Source: CAD feature listing. Evaluate the final solid. Frame: model axes, mm. Round coordinates to 2 decimals unless told otherwise and drop trailing zeros. Loops run counter-clockwise (first coordinate to the right, second up) from the corner with the lowest first, then second, coordinate; pieces in that order, holes last. Notation, with made-up numbers: (-22.5, -14.5) - (34.5, -14.5) arc R13 cw to (34.5, 1.5) - close; hole circle Ø7 at (41, 2). An arc over 180 degrees is marked (long way). One line per question, with ' | ' between items. Start each with the question number.
1. Ray query, line 1 (X direction, y = 303, z = 6.75); line 2 (X direction, y = 427.5, z = 3.2); line 3 (Y direction, x = 309, z = 9.5). Return the intervals inside material, ascending.
2. Cut plane B-B (y = 55). Return loops of the section in (x, z).
3. Pin query (flat end, axial travel): pin 1 (5 mm diameter, centred on y = 187, z = 4.5, fed in from +X); pin 2 (4 mm diameter, centred on x = 111, y = 303, fed in from -Z); pin 3 (3 mm diameter, centred on y = 393.5, z = 6, fed in from +X); pin 4 (2.5 mm diameter, centred on x = 314, z = 7, fed in from +Y). Return the tip coordinate at first contact, or that it passes through.
4. Cut plane D-D (z = 2.5). Return loops of the section in (x, y).
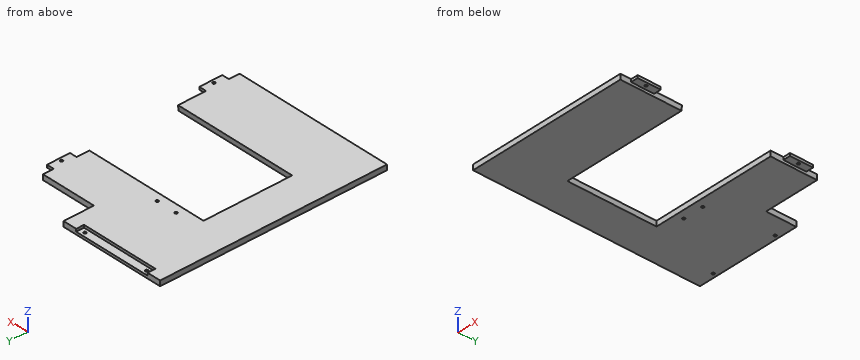
Autodesk Inventor part; units mm, degrees
ref_plane "YZ Plane" through (0, 0, 0) normal (1, 0, 0) x (0, 1, 0)
ref_plane "XZ Plane" through (0, 0, 0) normal (0, 1, 0) x (-1, 0, 0)
ref_plane "XY Plane" through (0, 0, 0) normal (0, 0, 1) x (1, 0, 0)
sketch "Sketch1" plane through (0, 0, 0) normal (0, 0, 1) x (1, 0, 0)
  line L0 (0, 0) -> (620, 0)
  line L1 (620, 0) -> (620, 620)
  line L2 (620, 620) -> (0, 620)
  line L3 (0, 620) -> (0, 0)
  line L4 (203, 491) -> (417, 491)
  line L5 (417, 491) -> (417, 377)
  line L6 (417, 377) -> (203, 377)
  line L7 (203, 377) -> (203, 491)
  point P0 (310, 491)
  point P1 (310, 620)
  dimension "d0" = 620
  dimension "d1" = 620
  dimension "d2" = 214
  dimension "d3" = 114
  dimension "d4" = 129
extrude "Extrusion1" add sketch "Sketch1" along normal blind 10
sketch "Sketch2" plane through (0, 0, 10) normal (0, 0, 1) x (1, 0, 0)
  line L0 (0, 0) -> (310, 0)
  line L1 (310, 0) -> (310, 435)
  line L2 (310, 435) -> (0, 435)
  line L3 (0, 435) -> (0, 0)
  line L4 (620, 620) -> (0, 620)
  line L5 (0, 435) -> (620, 435)
  line L6 (620, 435) -> (620, 620)
  line L7 (620, 620) -> (0, 620)
  line L8 (0, 620) -> (0, 435)
  line L9 (310, 435) -> (620, 435)
  line L10 (620, 435) -> (620, 0)
  line L11 (620, 0) -> (310, 0)
  line L12 (310, 0) -> (310, 435)
  point P0 (310, 620)
  dimension "d7" = 435
extrude "Extrusion2" cut sketch "Sketch2" against normal through all contours L1 L5 L10 L11 | L8 L4 L6 L5 L2
sketch "Sketch3" plane through (0, 0, 10) normal (0, 0, 1) x (1, 0, 0)
  line L0 (310, 0) -> (310, 377)
  line L1 (310, 356.5) -> (324, 356.5)
  line L2 (324, 356.5) -> (324, 312.5)
  line L3 (324, 312.5) -> (310, 312.5)
  line L4 (310, 312.5) -> (310, 356.5)
  circle A0 centre (317.5, 334.5) radius 2.5
  line L5 (203, 377) -> (310, 377)
  line L6 (310, 20.5) -> (324, 20.5)
  line L7 (324, 20.5) -> (324, 64.5)
  line L8 (324, 64.5) -> (310, 64.5)
  line L9 (310, 64.5) -> (310, 20.5)
  circle A1 centre (317.5, 42.5) radius 2.5
  line L10 (0, 0) -> (310, 0)
  dimension "d32" = 14
  dimension "d33" = 44
  dimension "d34" = 5
  dimension "d35" = 7.5
  dimension "d36" = 22
  dimension "d37" = 20.5
  dimension "d38" = 14
  dimension "d39" = 44
  dimension "d40" = 5
  dimension "d41" = 7.5
  dimension "d42" = 20.5
  dimension "d43" = 22
extrude "Extrusion3" add sketch "Sketch3" against normal blind 5
sketch "Sketch4" plane through (0, 0, 10) normal (0, 0, 1) x (1, 0, 0)
  line L0 (203, 435) -> (0, 435)
  line L1 (26.5, 435) -> (176.5, 435)
  line L2 (176.5, 435) -> (176.5, 420)
  line L3 (176.5, 420) -> (26.5, 420)
  line L4 (26.5, 420) -> (26.5, 435)
  point P0 (0, 0)
  point P1 (101.5, 435)
  dimension "d18" = 150
  dimension "d19" = 15
extrude "Extrusion4" cut sketch "Sketch4" against normal blind 5
sketch "Sketch5" plane through (0, 0, 5) normal (0, 0, 1) x (1, 0, 0)
  circle A0 centre (36.5, 427.5) radius 2.5
  circle A1 centre (166.5, 427.5) radius 2.5
  line L0 (26.5, 420) -> (26.5, 435)
  line L1 (176.5, 435) -> (176.5, 420)
  point P0 (0, 0)
  point P1 (26.5, 427.5)
  dimension "d22" = 5
  dimension "d23" = 5
  dimension "d24" = 10
  dimension "d25" = 10
extrude "Extrusion5" cut sketch "Sketch5" against normal through all
sketch "Sketch6" plane through (0, 0, 0) normal (0, 0, -1) x (-1, 0, 0)
  line L0 (-310, 64.5) -> (-310, 312.5)
  line L1 (-310, 288) -> (-70, 288)
  line L2 (-70, 288) -> (-70, 118)
  line L3 (-70, 118) -> (-310, 118)
  line L4 (-310, 118) -> (-310, 288)
  line L5 (-310, 312.5) -> (-324, 312.5)
  point P0 (0, 0)
  dimension "d44" = 240
  dimension "d45" = 170
  dimension "d55" = 24.5
extrude "Extrusion6" cut sketch "Sketch6" against normal through all
sketch "Sketch7" plane through (0, 0, 0) normal (0, 0, -1) x (-1, 0, 0)
  circle A0 centre (-111, 303) radius 2.5
  circle A1 centre (-151, 303) radius 2.5
  line L0 (-70, 288) -> (-70, 118)
  line L1 (-310, 288) -> (-70, 288)
  point P0 (0, 0)
  dimension "d48" = 5
  dimension "d49" = 5
  dimension "d50" = 40
  dimension "d51" = 41
  dimension "d52" = 15
extrude "Extrusion7" cut sketch "Sketch7" against normal through all
chamfer "Chamfer1" distance 10 angle 5 1 edges at (190, 118, 0) measured on face at (150, 118, 3.3333)
properties part number "TC001b" material "ABS Plastic"
Answers follow:
1) line 1: x = 0 to 108.5, 113.5 to 148.5, 153.5 to 310 | line 2: x = 0 to 34, 39 to 164, 169 to 203 | line 3: y = 0 to 117.96, 288 to 377
2) outline: (0, 0) - (310, 0) - (310, 5) - (324, 5) - (324, 10) - (0, 10) - close
3) pin 1: stops at x = 70 | pin 2: passes through | pin 3: stops at x = 203 | pin 4: stops at y = 356.5
4) outline: (0, 0) - (310, 0) - (310, 117.34) - (70, 117.34) - (70, 288) - (310, 288) - (310, 377) - (203, 377) - (203, 435) - (0, 435) - close; hole circle Ø5 at (36.5, 427.5); hole circle Ø5 at (111, 303); hole circle Ø5 at (151, 303); hole circle Ø5 at (166.5, 427.5)
